Autodesk Inventor part; units mm, degrees
ref_plane "YZ Plane" through (0, 0, 0) normal (1, 0, 0) x (0, 1, 0)
ref_plane "XZ Plane" through (0, 0, 0) normal (0, 1, 0) x (-1, 0, 0)
ref_plane "XY Plane" through (0, 0, 0) normal (0, 0, 1) x (1, 0, 0)
sketch "Sketch1" plane through (0, 0, 0) normal (0, 0, 1) x (1, 0, 0)
  line L0 (0, 117.6) -> (0, -117.6)
  line L1 (-194.6, 0) -> (194.6, 0)
  line L2 (-89, 84) -> (89, 84)
  line L3 (139, 34) -> (139, -34)
  line L4 (89, -84) -> (-89, -84)
  line L5 (-139, -34) -> (-139, 34)
  circle A0 centre (-95, 0) radius 25
  circle A1 centre (95, 0) radius 25
  circle A2 centre (0, 0) radius 45
  line L6 (-89, 84) -> (-139, 34)
  line L7 (89, 84) -> (139, 34)
  line L8 (139, -34) -> (89, -84)
  line L9 (-89, -84) -> (-139, -34)
  point P0 (-139, 84)
  point P1 (139, 84)
  point P2 (-139, -84)
  point P3 (139, -84)
  dimension "d0" = 278
  dimension "d1" = 168
  dimension "d8" = 50
  dimension "d9" = 190
  dimension "d10" = 95
  dimension "d11" = 90
  dimension "d12" = 50
  dimension "d13" = 50
  dimension "d14" = 50
  dimension "d15" = 50
  dimension "d16" = 50
  dimension "d17" = 50
  dimension "d18" = 50
  dimension "d19" = 50
extrude "Extrusion2" add sketch "Sketch1" against normal blind 10 contours L2 L7 L3 L1 A1 A2 L0 | L0 A2 L1 A0 L5 L6 L2 | L1 A1 L3 L8 L4 L0 A2 | A2 L0 L4 L9 L5 L1 A0
sketch "Sketch2" plane through (0, 0, 0) normal (0, 0, 1) x (1, 0, 0)
  line L0 (-139, -34) -> (-89, -84)
  line L1 (-89, -84) -> (89, -84)
  line L2 (89, -84) -> (139, -34)
  line L3 (139, -34) -> (139, 34)
  line L4 (139, 34) -> (89, 84)
  line L5 (89, 84) -> (-89, 84)
  line L6 (-89, 84) -> (-139, 34)
  line L7 (-139, 34) -> (-139, -34)
  circle A0 centre (-95, 0) radius 25
  circle A1 centre (0, 0) radius 45
  circle A2 centre (95, 0) radius 25
  line L8 (-35, 36.0385) -> (35, 36.0385)
  line L9 (35, 36.0385) -> (35, -36.0385)
  line L10 (35, -36.0385) -> (-35, -36.0385)
  line L11 (-35, -36.0385) -> (-35, 36.0385)
  line L12 (0, 117.6) -> (0, -117.6)
  line L13 (-194.6, 0) -> (194.6, 0)
  dimension "d22" = 70
hole "Hole1" at (-35, 36.0385, 0) at (35, 36.0385, 0) at (-35, -36.0385, 0) at (35, -36.0385, 0) direction (0, 0, -1) diameter 6.647 end through all
chamfer "Chamfer2" distance 0.5 angle 45 8 edges at (-35, -32.715, -10) (35, -32.715, -10) (-35, 39.362, -10) (35, 39.362, -10) (-35, -32.715, 0) (35, -32.715, 0) (-35, 39.362, 0) (35, 39.362, 0)
properties part number "SlipersLåda 211018004-1"
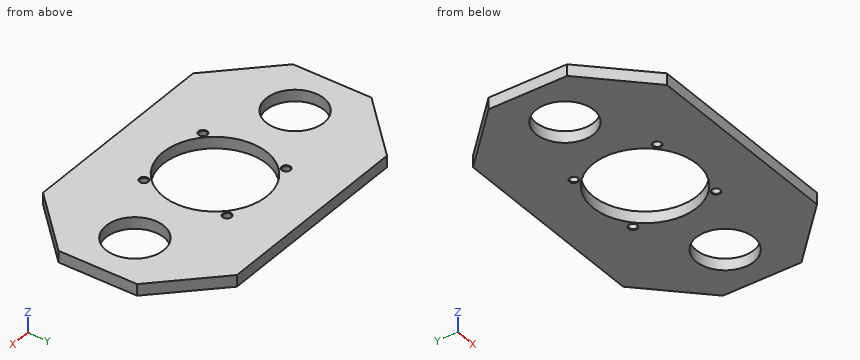
Geometry: final body of the model. Coordinates: model frame, mm. Coordinates: 2 decimals unless noted, no trailing zeros. Order: outer loops, then holes, each group sorted by start corner. A loop starts at its lowest first (then second) coordinate and runs counter-clockwise, first axis right, second up. Notation, with made-up numbers: (88, -29.5) -> (121, -29.5) arc R18 ccw to (121, 1.5) -> close; hole circle Ø1 at (-35, -12.75). An arc over 180 degrees is marked (long way). Use CSV: the item, a comma, the result in double quotes.
1) Section B-B on x = 0. Output: boundary loops of the cut face in (y, z), then the cut area to 3 significant figures.
Findings:
outline,"(-84, -10) -> (-45, -10) -> (-45, 0) -> (-84, 0) -> close; (45, -10) -> (84, -10) -> (84, 0) -> (45, 0) -> close"
area,"780 mm^2"
2) Section D-D on x = 35. Output: boundary loops of the cut face in (y, z) (3 decimals).
Findings:
outline,"(-84, -10) -> (-39.862, -10) -> (-39.362, -9.5) -> (-39.362, -0.5) -> (-39.862, 0) -> (-84, 0) -> close; (-32.715, -9.5) -> (-32.215, -10) -> (-28.284, -10) -> (-28.284, 0) -> (-32.215, 0) -> (-32.715, -0.5) -> close; (28.284, -10) -> (32.215, -10) -> (32.715, -9.5) -> (32.715, -0.5) -> (32.215, 0) -> (28.284, 0) -> close; (39.362, -9.5) -> (39.862, -10) -> (84, -10) -> (84, 0) -> (39.862, 0) -> (39.362, -0.5) -> close"
3) Pin query (flat end, axial travel): pin 1 Ø2 at (y, z) = (53, -1) entering from +X; pin 2 Ø4 at (x, y) = (-35, -36.04) entering from +Z; pin 3 Ø6 at (y, z) = (-43.5, -2) entering from +X; pin 4 Ø6 at (y, z) = (-50, -4) entering from +X. Return the tip coordinate at first contact, or that it passes through.
Findings:
pin 1,"stops at x = 121"
pin 2,"passes through"
pin 3,"stops at x = 132.5"
pin 4,"stops at x = 126"
4) Section A-A on y = 0. Output: boundary loops of the cut face in (x, z).
Findings:
outline,"(-139, -10) -> (-120, -10) -> (-120, 0) -> (-139, 0) -> close; (-70, -10) -> (-45, -10) -> (-45, 0) -> (-70, 0) -> close; (45, -10) -> (70, -10) -> (70, 0) -> (45, 0) -> close; (120, -10) -> (139, -10) -> (139, 0) -> (120, 0) -> close"
5) Line query: line 1 (X direction, y = 0, z = -4); line 2 (X direction, y = 20.5, z = -4); line 3 (Y direction, x = -95, z = -5). Output: solid intervals per line, ascending.
Findings:
line 1,"x = -139 to -120, -70 to -45, 45 to 70, 120 to 139"
line 2,"x = -139 to -109.31, -80.69 to -40.06, 40.06 to 80.69, 109.31 to 139"
line 3,"y = -78 to -25, 25 to 78"
6) Section C-C on z = -2.25. Output: boundary loops of the cut face in (x, y) (1 decimal).
Findings:
outline,"(-139, -34) -> (-89, -84) -> (89, -84) -> (139, -34) -> (139, 34) -> (89, 84) -> (-89, 84) -> (-139, 34) -> close; hole circle Ø50 at (-95, 0); hole circle Ø90 at (0, 0); hole circle Ø6.6 at (-35, -36); hole circle Ø6.6 at (-35, 36); hole circle Ø6.6 at (35, -36); hole circle Ø6.6 at (35, 36); hole circle Ø50 at (95, 0)"
